Input: part model. Units: mm. Frame: model coordinates. Face numbers are marked on the shaded views. A direction names the side the tool comes from. Round coordinates to 2 decimals unless told otherwise and drop trailing zeros. Write each loop counter-clockwise with the first axis right and the second up, starting at its lowest first coordinate (ties: lowest second). Pieces come first, ordered by that corner, then holes. Notation, with made-up numbers: (43.25, 85.5) - (63.25, 85.5) arc R28 cw to (63.25, 106.5) - close; hole circle Ø2 at (30, -20.75). An arc over 180 degrees is marked (long way). One line per item, written item: value. Start each with the question number.
```python
from build123d import *

# Parameters (mm, degrees)
F0_W      = 1833.88
F0_H      = 1295.4
F0_W_2    = 1757.68
F0_H_2    = 1219.2
F1_DEPTH  = 508
F2_R      = 50.8
F3_R      = 50.8
F4_R      = 50.8
F5_R      = 50.8
F6_R      = 25.4
F8_DEPTH  = 50.8
F7_R      = 12.7
F9_DEPTH  = 50.8
F10_R     = 27.856725
F11_DEPTH = 50.8


with BuildPart() as f1:
    # F0 (on Top) → F1 (new body)
    with BuildSketch(Plane.XY):
        with Locations((878.84, 609.6)):
            Rectangle(F0_W, F0_H)
        with Locations((878.84, 609.6)):
            Rectangle(F0_W_2, F0_H_2, mode=Mode.SUBTRACT)
    extrude(amount=F1_DEPTH)

    # F2
    f2_edges = [f1.edges().sort_by_distance(p)[0] for p in [
        (1757.68, 1219.2, 254),
    ]]
    fillet(f2_edges, radius=F2_R)

    # F3
    f3_edges = [f1.edges().sort_by_distance(p)[0] for p in [
        (0, 1219.2, 254),
    ]]
    fillet(f3_edges, radius=F3_R)

    # F4
    f4_edges = [f1.edges().sort_by_distance(p)[0] for p in [
        (1757.68, 0, 254),
    ]]
    fillet(f4_edges, radius=F4_R)

    # F5
    f5_edges = [f1.edges().sort_by_distance(p)[0] for p in [
        (0, 0, 254),
    ]]
    fillet(f5_edges, radius=F5_R)

    # F6 (on face) → F8 (cut)
    with BuildSketch(Plane(origin=(-38.1, 0, 0), x_dir=(0, -1, 0), z_dir=(-1, 0, 0))):
        with Locations((-604.977846, 41.91)):
            Circle(F6_R)
        with Locations((-706.577846, 41.91)):
            Circle(F6_R)
    extrude(amount=-F8_DEPTH, mode=Mode.SUBTRACT)

    # F7 (on face) → F9 (cut)
    with BuildSketch(Plane(origin=(-38.1, 0, 0), x_dir=(0, -1, 0), z_dir=(-1, 0, 0))):
        with Locations((-393.7, 16.51)):
            Circle(F7_R)
        with Locations((-825.5, 16.51)):
            Circle(F7_R)
    extrude(amount=-F9_DEPTH, mode=Mode.SUBTRACT)

    # F10 (on face) → F11 (cut)
    with BuildSketch(Plane.YZ.offset(1795.78)):
        with Locations((609.6, 41.91)):
            Circle(F10_R)
    extrude(amount=-F11_DEPTH, mode=Mode.SUBTRACT)


solid = f1.part
```
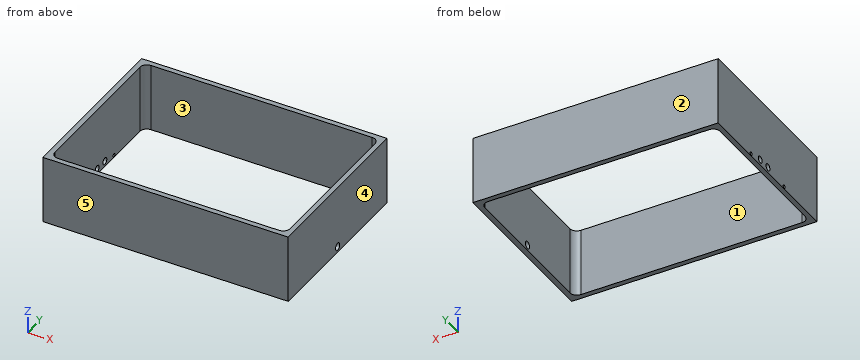
Q1. Cut plane C-C, the plane y = 924. Output: boundary loops of the cut face in (x, z).
Q2. Cut plane A-A, the plane x = 128.5. Output: boundary loops of the cut face in (y, z), and give its area (3 significant figures).
Q3. Pull-direction query (X, two-part tool) for the marked faces 3, 4 and 5; classes: pulls with the +X half, pulls with the -X half, needs draft (parallel to the pull), parting line crosses it, or undercut.
Q4. Material intervals for probe 1 along X at (y, z) = (87, 60); probe 2 along Z at (x, y) = (-29, 393.7); probe 3 along Z at (x, y) = (1786, 609), sorted ascending. Write a range as from..to.
Q5. Cut plane B-B, the plane z = 179. Output: boundary loops of the cut face in (x, y).
Q6. Access query for the marked faces 1 and 2. Directions: +Z, -Z, +X, -X, +Y, -Y. A direction counts if a zero-diameter tool reaches every point of the face in a straight line with its end or side. Return the directions, or none.
Q7. Cut plane D-D, the plane y = 609.6. Output: boundary loops of the cut face in (x, z).
Q8. Contact query for a flat-ended pin moving along its axis: pin 1 Ø15 at (y, z) = (825.5, 16.51) entering from -X. Output: stop coordinate, or through.
A:
1. outline: (-38.1, 0) - (0, 0) - (0, 508) - (-38.1, 508) - close; (1757.68, 0) - (1795.78, 0) - (1795.78, 508) - (1757.68, 508) - close
2. outline: (-38.1, 0) - (0, 0) - (0, 508) - (-38.1, 508) - close; (1219.2, 0) - (1257.3, 0) - (1257.3, 508) - (1219.2, 508) - close
2. area: 38,700 mm²
3. face 3: undercut
3. face 4: pulls with the +X half
3. face 5: needs draft
4. probe 1: x = -38.1..0, 1757.68..1795.78
4. probe 2: z = 0..3.81, 29.21..508
4. probe 3: z = 0..14.06, 69.76..508
5. outline: (-38.1, -38.1) - (1795.78, -38.1) - (1795.78, 1257.3) - (-38.1, 1257.3) - close; hole (0, 50.8) arc R50.8 ccw to (50.8, 0) - (1706.88, 0) arc R50.8 ccw to (1757.68, 50.8) - (1757.68, 1168.4) arc R50.8 ccw to (1706.88, 1219.2) - (50.8, 1219.2) arc R50.8 ccw to (0, 1168.4) - close
6. face 1: +Z, -Z
6. face 2: +Z, -Z, +X, -X, +Y
7. outline: (-38.1, 0) - (0, 0) - (0, 16.93) - (-38.1, 16.93) - close; (-38.1, 66.89) - (0, 66.89) - (0, 508) - (-38.1, 508) - close; (1757.68, 0) - (1795.78, 0) - (1795.78, 14.05) - (1757.68, 14.05) - close; (1757.68, 69.77) - (1795.78, 69.77) - (1795.78, 508) - (1757.68, 508) - close
8. pin 1: stops at x = 1757.68
